Check sheet for the modelled part. Datum: model origin and axes. Units: mm. A direction names the side the tool comes from. Give positions to 0.01 mm unless a question says otherwise; leave off trailing zeros. Write each loop counter-clockwise with the first axis right and the second up, starting at its lowest first coordinate (ties: lowest second). Pieces come first, ordered by that corner, then holes. Notation, with made-up numbers: M 32.25,-30.5 L 51.25,-30.5 A26 cw 51.25,-1.5 Z; hole C 63.5,80 d1. An arc over 180 degrees is marked long. Write item = value, one per line. Start each with the question number.
1) Cross-section at B-B, the plane x = 14.7. Record the cut outline in (y, z).
2) Mould release check, pull along X, two halves, no side actions. Record for faces 1 (the flat face through (25.4, 0, 94)), 2 (the flat face through (29.4, 0, 2)), 3 (the cylindrical face through (27, 0, 109)): released by +X, released by -X, zero draft, split by the parting line, or undercut.
3) Cross-section at C-C, the plane z = 94.5. Record the cut outline in (x, y), plus the area to 3 significant figures.
4) Access from +Z, -Z, +X, -X, +Y, -Y to the whole of each face (thin tool, end or side, straight path). Record for faces 4 (the flat face through (4, 0, 94)), 5 (the flat face through (4, 0, -94)), 6 (the cylindrical face through (14.5, -0.1, 75)).
5) Go/stop test with flat-tipped pins: pin 1 (1 mm diameter, centred on x = 19, y = -3, fed in from -Z); pin 2 (7 mm diameter, centred on y = 0, z = 57, fed in from +X); pin 3 (7.5 mm diameter, centred on x = 19.5, y = 2.5, fed in from +Z). Record where each tip stops, or that it passes through.
6) Cross-section at D-D, the plane y = 0. Give the number of separate pieces and of enclosed holes in the cut face, plus the area to 3 significant figures.
7) Cross-section at A-A, the plane z = 57. Record the cut outline in (x, y).
8) Scan lines: line 1 along X through (y, z) = (-1.5, 34.5); line 2 along Z through (x, y) = (27, -2); line 3 along X through (y, z) = (6.75, -96). Record each from-to range of solid material in increasing order. Write a range as [from, to].
```python
from build123d import *

# Parameters (mm, degrees)
EXTRUDE_1_DEPTH     = 29.4
SKETCH_3_W          = 21.4
SKETCH_3_H          = 30
CUT_EXTRUDE_1_DEPTH = 118.241673478
SKETCH_4_R          = 4
SKETCH_4_R_2        = 5
CUT_EXTRUDE_2_DEPTH = 117.519783728
CUT_EXTRUDE_3_DEPTH = 118.241673478
SKETCH_6_R          = 3
CUT_EXTRUDE_4_DEPTH = 117.519783728


with BuildPart() as part:
    # 草图2 → 凸台-拉伸1 (new body)
    with BuildSketch(Plane(origin=(0, 0, 0), x_dir=(0, 0, -1), z_dir=(1, 0, 0))):
        with BuildLine():
            Line((-105, -7.5), (105, -7.5))
            ThreePointArc((105, -7.5), (112.5, 0), (105, 7.5))
            Line((105, 7.5), (-105, 7.5))
            ThreePointArc((-105, 7.5), (-112.5, 0), (-105, -7.5))
        make_face()
    extrude(amount=EXTRUDE_1_DEPTH)

    # 草图3 → 切除-拉伸1 (cut, through all)
    with BuildSketch(Plane(origin=(0, 7.5, 0), x_dir=(1, 0, 0), z_dir=(0, 1, 0))):
        with Locations((14.7, -97.5)):
            Rectangle(SKETCH_3_W, SKETCH_3_H)
        with Locations((14.7, 97.5)):
            Rectangle(SKETCH_3_W, SKETCH_3_H)
    extrude(amount=-CUT_EXTRUDE_1_DEPTH, mode=Mode.SUBTRACT)

    # 草图4 → 切除-拉伸2 (cut, through all)
    with BuildSketch(Plane(origin=(29.4, 0, 0), x_dir=(0, 0, -1), z_dir=(1, 0, 0))):
        with Locations((-105, 0)):
            Circle(SKETCH_4_R)
        with Locations((105, 0)):
            Circle(SKETCH_4_R_2)
    extrude(amount=-CUT_EXTRUDE_2_DEPTH, mode=Mode.SUBTRACT)

    # 草图5 → 切除-拉伸3 (cut, through all)
    with BuildSketch(Plane.XZ.offset(7.5)):
        with BuildLine():
            Line((24.7, 65), (24.7, -65))
            ThreePointArc((24.7, -65), (14.7, -75), (4.7, -65))
            Line((4.7, -65), (4.7, 65))
            ThreePointArc((4.7, 65), (14.7, 75), (24.7, 65))
        make_face()
    extrude(amount=-CUT_EXTRUDE_3_DEPTH, mode=Mode.SUBTRACT)

    # 草图6 → 切除-拉伸4 (cut, through all)
    with BuildSketch(Plane.ZY):
        with Locations((57, 0)):
            Circle(SKETCH_6_R)
    extrude(amount=-CUT_EXTRUDE_4_DEPTH, mode=Mode.SUBTRACT)


solid = part.part
```
Reply:
q1.outline = M -7.5,-82.5 L 7.5,-82.5 L 7.5,-75 L -7.5,-75 Z; M -7.5,75 L 7.5,75 L 7.5,82.5 L -7.5,82.5 Z
q2.face_1 = undercut
q2.face_2 = released by +X
q2.face_3 = zero draft
q3.outline = M 0,-7.5 L 4,-7.5 L 4,7.5 L 0,7.5 Z; M 25.4,-7.5 L 29.4,-7.5 L 29.4,7.5 L 25.4,7.5 Z
q3.area = 120 mm2
q4.face_4 = +Z, +Y, -Y
q4.face_5 = -Z, +Y, -Y
q4.face_6 = +Y, -Y
q5.pin_1 = -82.5
q5.pin_2 = 29.4
q5.pin_3 = 82.5
q6.separate_pieces = 6
q6.enclosed_holes = 0
q6.area = 2,220 mm2
q7.outline = M 0,-7.5 L 4.7,-7.5 L 4.7,-3 L 0,-3 Z; M 0,3 L 4.7,3 L 4.7,7.5 L 0,7.5 Z; M 24.7,-7.5 L 29.4,-7.5 L 29.4,-3 L 24.7,-3 Z; M 24.7,3 L 29.4,3 L 29.4,7.5 L 24.7,7.5 Z
q8.line_1 = [0, 4.7], [24.7, 29.4]
q8.line_2 = [-112.23, -109.58], [-100.42, 54.76], [59.24, 101.54], [108.46, 112.23]
q8.line_3 = [0, 4], [25.4, 29.4]
